```python
from build123d import *

# Parameters (mm, degrees)
F1_DEPTH = 20
F2_DEPTH = 4
F3_R     = 2.25
F4_DEPTH = 3
F3_W     = 8
F3_H     = 4.4
F3_W_2   = 3
F5_DEPTH = 1.5
F6_SIZE  = 1.49999
F8_SIZE  = 3


# Not quite as in the source:
# - a fillet or chamfer is up to 0.001 mm smaller than in the source, because OpenCascade refuses the exact size
# - a pattern or mirror of a feature is missing from the dataset's text; its kind, count and spacing are read off the source's solid


with BuildPart() as f1:
    # F0 (on Top) → F1 (new body)
    with BuildSketch(Plane.XY):
        Polygon((0, 20), (0, 0), (20, 0), (20, 3), (3, 3), (3, 20), align=None)
    extrude(amount=F1_DEPTH)

    # F0 (on Top) → F2 (join)
    with BuildSketch(Plane.XY):
        Polygon((3, 3), (20, 3), (3, 20), align=None)
    extrude(amount=F2_DEPTH)

    # F3 (on face) → F4 (cut, through all)
    with BuildSketch(Plane.XZ):
        with Locations((13, 10)):
            Circle(F3_R)
    f4 = extrude(amount=-F4_DEPTH, mode=Mode.SUBTRACT)

    # F4_copies: F4 across plane
    add(f4.mirror(Plane(origin=(0, 0, 0), x_dir=(-0.7071067812, -0.7071067812, 0), z_dir=(-0.7071067812, 0.7071067812, 0))), mode=Mode.SUBTRACT)

    # F3 (on face) → F5 (join)
    with BuildSketch(Plane.XZ):
        with Locations((4, 10)):
            Rectangle(F3_W, F3_H)
        with Locations((18.5, 10)):
            Rectangle(F3_W_2, F3_H)
    f5 = extrude(amount=F5_DEPTH)

    # F5_copies: F5 across plane
    add(f5.mirror(Plane(origin=(0, 0, 0), x_dir=(0.7071067812, 0.7071067812, 0), z_dir=(-0.7071067812, 0.7071067812, 0))))

    # F6 (size 1.5 in the source; OpenCascade refuses exactly that, so slightly less here)
    f6_edges = [f1.edges().sort_by_distance(p)[0] for p in [
        (4, -1.5, 7.8),
        (18.5, -1.5, 7.8),
        (-1.5, 4, 7.8),
        (-1.5, 18.5, 7.8),
    ]]
    chamfer(f6_edges, length=F6_SIZE)

    # F8
    f8_edges = [f1.edges().sort_by_distance(p)[0] for p in [
        (3, 3, 12),
    ]]
    chamfer(f8_edges, length=F8_SIZE)


solid = f1.part
```
Source: CAD feature listing. Evaluate the final solid. Frame: model axes, mm. A direction names the side the tool comes from. Give positions to 0.01 mm unless a question says otherwise; leave off trailing zeros. Loops run counter-clockwise (first coordinate to the right, second up) from the corner with the lowest first, then second, coordinate; pieces in that order, holes last. Notation, with made-up numbers: (7, 24.25) - (17, 24.25) arc R25 cw to (17, 60.25) - close; hole circle Ø1 at (44, 87). An arc over 180 degrees is marked (long way). Use CSV: the item, a comma, the result in double quotes. Start each with the question number.
1. Draft query along Z for faces 1 (the flat face through (-1, 18, 12.2)), 2 (the cylindrical face through (1.48, 11.34, 11.52)), 3 (the flat face through (12, 11, 2)). Return one class per face: +Z half, -Z half, draft (parallel to the pull), parting line (faces both ways), or undercut.
2. Section C-C (z = 10). Output: boundary loops of the cut face in (x, y), then the cut area to 4 significant figures.
3. Pin query (flat end, axial travel): pin 1 (4 mm diameter, centred on x = 13, z = 5, fed in from -Y); pin 2 (1.6 mm diameter, centred on x = 18.5, y = -1, fed in from +Z); pin 3 (5 mm diameter, centred on y = 13, z = 10, fed in from -X); pin 4 (4 mm diameter, centred on x = 13, z = 10, fed in from +Y). Return the tip coordinate at first contact, or that it passes through.
4. Section A-A (x = 13). Output: boundary loops of the cut face in (y, z), then the cut area to 3 significant figures.
5. Ray query, L1, parallel to Z at x = 13, y = 1.2; L2, parallel to Z at x = 10.75, y = 5; L3, parallel to Y at x = 6.25, z = 15. Return the intervals inside material, ascending.
6. Reachability of faces 4 (the flat face through (-1, 0, 10)), 5 (the flat face through (-1, 17, 10)), 6 (the flat face through (4, -1, 12.2)), 7 (the flat face through (8, -1, 10)), 8 (the flat face through (8, 8, 4)) from +Z, -Z, +X, -X, +Y, -Y: full face, straight path, thin tool, end or side. Return the list, or none.
Response:
1,face 1,"+Z half"
1,face 2,"undercut"
1,face 3,"draft"
2,outline,"(-1.5, 0) - (0, 0) - (0, -1.5) - (8, -1.5) - (8, 0) - (10.75, 0) - (10.75, 3) - (6, 3) - (3, 6) - (3, 10.75) - (0, 10.75) - (0, 8) - (-1.5, 8) - close; (-1.5, 17) - (0, 17) - (0, 15.25) - (3, 15.25) - (3, 20) - (-1.5, 20) - close; (15.25, 0) - (17, 0) - (17, -1.5) - (20, -1.5) - (20, 3) - (15.25, 3) - close"
2,area,"121.5 mm²"
3,pin 1,"y = 0"
3,pin 2,"z = 12.2"
3,pin 3,"x = 0"
3,pin 4,"through"
4,outline,"(0, 0) - (10, 0) - (10, 4) - (3, 4) - (3, 7.75) - (0, 7.75) - close; (0, 12.25) - (3, 12.25) - (3, 20) - (0, 20) - close"
4,area,"74.5 mm²"
5,L1,"0 to 7.75, 12.25 to 20"
5,L2,"0 to 4"
5,L3,"0 to 3"
6,face 4,"+Z, -Z, -X, -Y"
6,face 5,"+Z, -Z, -X"
6,face 6,"+Z, +X, -X, -Y"
6,face 7,"+Z, -Z, -Y"
6,face 8,"+Z, +X, +Y"
